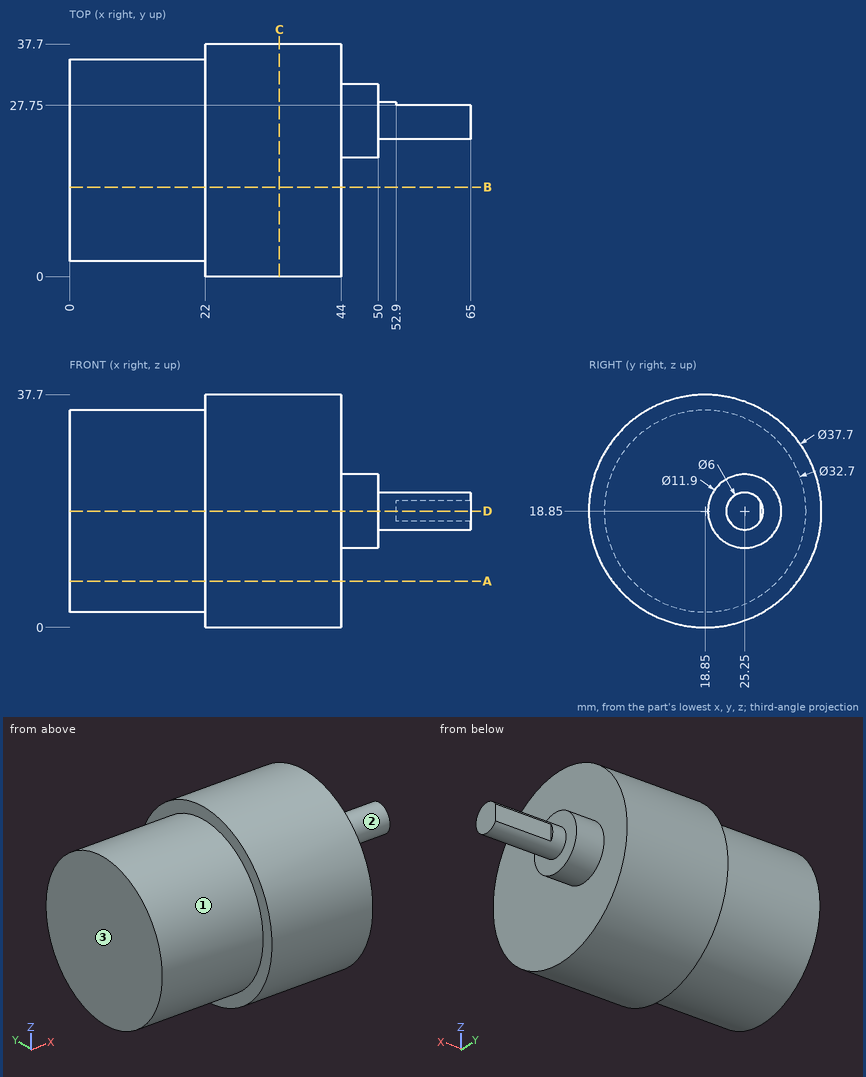
Geometry: see drawing. Coordinates: mm, zero at the bounding-box minimum. A direction names the side the tool comes from. Round coordinates to 2 decimals unless told otherwise and drop trailing zeros. Loops run counter-clockwise (first coordinate to the right, second up) from the corner with the lowest first, then second, coordinate; pieces in that order, holes last. Notation, with made-up numbers: M 80.5,-9.75 L 121.5,-9.75 A21 ccw 121.5,19.25 Z; hole C 11,45 d8. An arc over 180 degrees is marked long. Use a Markdown table: item, result. Add a question column.
1. Line query: line 1 (X direction, y = 14, z = 34.5); line 2 (X direction, y = 29.5, z = 27); line 3 (Z direction, x = 25.5, y = 19.5). Output: solid intervals per line, ascending.
2. Section query C-C on x = 34. Return the cut outline in (y, z), then the cut area to 3 significant figures.
3. Section query B-B on y = 14.5. Return the cut outline in (x, z), then the cut area to 3 significant figures.
4. Section query D-D on z = 18.85. Return the cut outline in (x, y), then the cut area to 3 significant figures.
5. Reachability of the marked faces 1, 2 and 3 from +Z, -Z, +X, -X, +Y, -Y: full face, straight path, thin tool, end or side. Return the list, or none.
6. Contact query for flat-ended pins moving along their axis: P1, Ø3.5, axis at x = 60, z = 18, coming from the +Y side; P2, Ø1, axis at x = 45.5, y = 12.5, coming from the -Z side; P3, Ø3, axis at x = 21.5, z = 23.5, coming from the -Y side; P4, Ø2, axis at x = 23.5, y = 28, coming from the -Z side. Output: stop coordinate, or through.
7. Section query A-A on z = 7.5. Return the cut outline in (x, y).
Reported:
| question | item | result |
|---|---|---|
| 1 | line 1 | x = 22 to 44 |
| 1 | line 2 | x = 0 to 44 |
| 1 | line 3 | z = 0.01 to 37.69 |
| 2 | outline | C 18.85,18.85 d37.7 |
| 2 | area | 1,120 mm² |
| 3 | outline | M 0,3.09 L 22,3.09 L 22,0.51 L 44,0.51 L 44,37.19 L 22,37.19 L 22,34.61 L 0,34.61 Z |
| 3 | area | 1,500 mm² |
| 4 | outline | M 0,2.5 L 22,2.5 L 22,0 L 44,0 L 44,19.3 L 50,19.3 L 50,22.25 L 65,22.25 L 65,27.75 L 52.9,27.75 L 52.9,28.25 L 50,28.25 L 50,31.2 L 44,31.2 L 44,37.7 L 22,37.7 L 22,35.2 L 0,35.2 Z |
| 4 | area | 1,700 mm² |
| 5 | face 1 | -X |
| 5 | face 2 | +X |
| 5 | face 3 | +Z, -Z, -X, +Y, -Y |
| 6 | P1 | stops at y = 27.75 |
| 6 | P2 | passes through |
| 6 | P3 | stops at y = 0.28 |
| 6 | P4 | stops at z = 1.85 |
| 7 | outline | M 0,7.08 L 22,7.08 L 22,3.8 L 44,3.8 L 44,33.9 L 22,33.9 L 22,30.62 L 0,30.62 Z |
